Work out the finished part from the listing and answer in its coordinate system (mm). Coordinates: 2 decimals unless noted, no trailing zeros. Answer as a JSON object with one key per item and string values. Group by question number.
1) Section A-A (z = 240.5) is taken. Count the separate pieces of the cut face and the enclosed holes in it, plus the area to 3 significant figures.
2) Each of these flat-tipped pins is pushed along its axis until it touches: P1, Ø1.2, axis at x = 14.5, z = 162, coming from the -Y side; P2, Ø6, axis at y = -0.5, z = 176, coming from the -X side; P3, Ø0.9, axis at x = 14.5, z = 153, coming from the +Y side. Where does it stop, or does it pass through?
3) Find the intervals of material crossed by line 1 along Y through (x, z) = (12.5, 157); line 2 along X through (y, z) = (-10.5, 112.5), in increasing order.
from build123d import *

# Parameters (mm, degrees)
SKETCH1_R                = 3.65
SKETCH1_W                = 4
SKETCH1_H                = 4
BOSS_EXTRUDE1_DEPTH      = 300
FILLET1_R                = 1
CIRPATTERN1_COUNT        = 4
FILLET1_OF_CIRPATTERN1_R = 1
CUT_EXTRUDE1_DEPTH       = 301.749064836
CUT_EXTRUDE2_DEPTH       = 301.749064836
CIRPATTERN2_COUNT        = 4


with BuildPart() as part:
    # Sketch1 → Boss-Extrude1 (new body)
    with BuildSketch(Plane.XY):
        with BuildLine():
            Line((5.1, 15), (13, 15))
            ThreePointArc((13, 15), (14.414213562, 14.414213562), (15, 13))
            Line((15, 13), (15, 5.1))
            Line((15, 5.1), (13.9, 5.1))
            Line((13.9, 5.1), (13.9, 4))
            Line((13.9, 4), (12.8, 4))
            Line((12.8, 4), (12.8, 8.25))
            Line((12.8, 8.25), (10.017766953, 8.25))
            Line((10.017766953, 8.25), (6, 4.232233047))
            Line((6, 4.232233047), (6, -6))
            Line((6, -6), (-6, -6))
            Line((-6, -6), (-6, 6))
            Line((-6, 6), (4.232233047, 6))
            Line((4.232233047, 6), (8.25, 10.017766953))
            Line((8.25, 10.017766953), (8.25, 12.8))
            Line((8.25, 12.8), (4, 12.8))
            Line((4, 12.8), (4, 13.9))
            Line((4, 13.9), (5.1, 13.9))
            Line((5.1, 13.9), (5.1, 15))
        make_face()
        Circle(SKETCH1_R, mode=Mode.SUBTRACT)
        with Locations((11.75, 11.75)):
            Rectangle(SKETCH1_W, SKETCH1_H, mode=Mode.SUBTRACT)
    boss_extrude1 = extrude(amount=BOSS_EXTRUDE1_DEPTH)

    # Fillet1
    fillet1_edges = [part.edges().sort_by_distance(p)[0] for p in [
        (9.75, 13.75, 150),
        (9.75, 9.75, 150),
        (13.75, 9.75, 150),
        (13.75, 13.75, 150),
    ]]
    fillet(fillet1_edges, radius=FILLET1_R)

    # CirPattern1: Boss-Extrude1 ×4 about axis
    cirpattern1_axis = Axis((0, 0, 0), (0, 0, 1))
    for i in range(1, CIRPATTERN1_COUNT):
        add(boss_extrude1.rotate(cirpattern1_axis, i * 360 / CIRPATTERN1_COUNT))

    # Fillet1 of CirPattern1
    fillet1_of_cirpattern1_edges = [part.edges().sort_by_distance(p)[0] for p in [
        (-13.75, 9.75, 150),
        (-9.75, 9.75, 150),
        (-9.75, 13.75, 150),
        (-13.75, 13.75, 150),
        (-9.75, -13.75, 150),
        (-9.75, -9.75, 150),
        (-13.75, -9.75, 150),
        (-13.75, -13.75, 150),
        (13.75, -9.75, 150),
        (9.75, -9.75, 150),
        (9.75, -13.75, 150),
        (13.75, -13.75, 150),
    ]]
    fillet(fillet1_of_cirpattern1_edges, radius=FILLET1_OF_CIRPATTERN1_R)

    # Sketch2 → Cut-Extrude1 (cut, through all)
    with BuildSketch(Plane(origin=(0, 0, 0), x_dir=(-1, 0, 0), z_dir=(0, 0, -1))):
        Polygon((0, 5.5), (-0.5, 6), (0.5, 6), align=None)
    cut_extrude1 = extrude(amount=-CUT_EXTRUDE1_DEPTH, mode=Mode.SUBTRACT)

    # Sketch3 → Cut-Extrude2 (cut, through all)
    with BuildSketch(Plane(origin=(0, 0, 0), x_dir=(-1, 0, 0), z_dir=(0, 0, -1))):
        with BuildLine():
            Line((-1.775079755, 3.189293317), (-2.828427125, 4.242640687))
            Line((-2.828427125, 4.242640687), (-4.242640687, 2.828427125))
            Line((-4.242640687, 2.828427125), (-3.189293317, 1.775079755))
            ThreePointArc((-3.189293317, 1.775079755), (-2.580939751, 2.580939751), (-1.775079755, 3.189293317))
        make_face()
    cut_extrude2 = extrude(amount=-CUT_EXTRUDE2_DEPTH, mode=Mode.SUBTRACT)

    # CirPattern2: Cut-Extrude1, Cut-Extrude2 ×4 about axis
    cirpattern2_axis = Axis((0, 0, 0), (0, 0, 1))
    add([cut_extrude1.rotate(cirpattern2_axis, i * 360 / CIRPATTERN2_COUNT) for i in range(1, CIRPATTERN2_COUNT)], mode=Mode.SUBTRACT)
    add([cut_extrude2.rotate(cirpattern2_axis, i * 360 / CIRPATTERN2_COUNT) for i in range(1, CIRPATTERN2_COUNT)], mode=Mode.SUBTRACT)


solid = part.part
Report:
{
 "1": {"separate pieces": "1", "enclosed holes": "5", "area": "318 mm²"},
 "2": {"P1": "stops at y = -14.79", "P2": "stops at x = -6", "P3": "stops at y = 14.7"},
 "3": {"line 1": "y = -15 to -13.75, -9.75 to -8.25, 8.25 to 9.75, 13.75 to 15", "line 2": "x = -15 to -13.72, -9.78 to -8.25, 8.25 to 9.78, 13.72 to 15"}
}
